Model file for the job. Use its own axes, mm. A direction names the side the tool comes from. Coordinates: 2 decimals unless noted, no trailing zeros. Order: outer loops, then holes, each group sorted by start corner. A loop starts at its lowest first (then second) coordinate and runs counter-clockwise, first axis right, second up.
from build123d import *

# Parameters (mm, degrees)
F0_W     = 38
F0_H     = 69
F0_W_2   = 28
F0_H_2   = 28
F0_H_3   = 1
F0_W_3   = 1
F1_DEPTH = 5
F2_DEPTH = 25
F3_DEPTH = 4
F4_R     = 4.99999


# Not quite as in the source:
# - a fillet or chamfer is up to 0.001 mm smaller than in the source, because OpenCascade refuses the exact size


with BuildPart() as f1:
    # F0 (on Front) → F1 (new body)
    with BuildSketch(Plane.XZ):
        Rectangle(F0_W, F0_H)
        Polygon((-15, 0.5), (-15, 1.5), (-15, 30.5), (15, 30.5), (15, 1.5), (15, 0.5), (15, -0.5), (15, -1.5), (15, -30.5), (-15, -30.5), (-15, -1.5), (-15, -0.5), align=None, mode=Mode.SUBTRACT)
        with Locations((0, 15.5)):
            Rectangle(F0_W_2, F0_H_2)
        with Locations((0, -15.5)):
            Rectangle(F0_W_2, F0_H_2)
        Polygon((-14, -29.5), (-14, -1.5), (-15, -1.5), (-15, -30.5), (15, -30.5), (15, -1.5), (14, -1.5), (14, -29.5), align=None)
        Polygon((-14, 1.5), (-14, 29.5), (14, 29.5), (14, 1.5), (15, 1.5), (15, 30.5), (-15, 30.5), (-15, 1.5), align=None)
        with Locations((0, 1)):
            Rectangle(F0_W_2, F0_H_3)
        with Locations((0, -1)):
            Rectangle(F0_W_2, F0_H_3)
        Rectangle(F0_W_2, F0_H_3)
        with Locations((-14.5, 1)):
            Rectangle(F0_W_3, F0_H_3)
        with Locations((-14.5, 0)):
            Rectangle(F0_W_3, F0_H_3)
        with Locations((-14.5, -1)):
            Rectangle(F0_W_3, F0_H_3)
        with Locations((14.5, 1)):
            Rectangle(F0_W_3, F0_H_3)
        with Locations((14.5, 0)):
            Rectangle(F0_W_3, F0_H_3)
        with Locations((14.5, -1)):
            Rectangle(F0_W_3, F0_H_3)
    extrude(amount=F1_DEPTH)

    # F0 (on Front) → F2 (cut)
    with BuildSketch(Plane.XZ):
        with Locations((0, 15.5)):
            Rectangle(F0_W_2, F0_H_2)
        with Locations((0, -15.5)):
            Rectangle(F0_W_2, F0_H_2)
    extrude(amount=F2_DEPTH, mode=Mode.SUBTRACT)

    # F0 (on Front) → F3 (cut)
    with BuildSketch(Plane.XZ):
        Polygon((-14, 1.5), (-14, 29.5), (14, 29.5), (14, 1.5), (15, 1.5), (15, 30.5), (-15, 30.5), (-15, 1.5), align=None)
        with Locations((14.5, 1)):
            Rectangle(F0_W_3, F0_H_3)
        with Locations((0, 1)):
            Rectangle(F0_W_2, F0_H_3)
        with Locations((-14.5, 1)):
            Rectangle(F0_W_3, F0_H_3)
        Polygon((-14, -29.5), (-14, -1.5), (-15, -1.5), (-15, -30.5), (15, -30.5), (15, -1.5), (14, -1.5), (14, -29.5), align=None)
        with Locations((14.5, -1)):
            Rectangle(F0_W_3, F0_H_3)
        with Locations((0, -1)):
            Rectangle(F0_W_2, F0_H_3)
        with Locations((-14.5, -1)):
            Rectangle(F0_W_3, F0_H_3)
    extrude(amount=F3_DEPTH, mode=Mode.SUBTRACT)

    # F4 (radius 5 in the source; OpenCascade refuses exactly that, so slightly less here)
    f4_edges = [f1.edges().sort_by_distance(p)[0] for p in [
        (-19, -5, 0),
        (0, -5, 34.5),
        (19, -5, 0),
        (0, -5, -34.5),
    ]]
    fillet(f4_edges, radius=F4_R)


solid = f1.part
Q1. Cut at B-B, the plane x = 4.5. Count the separate pieces of the cut face and the enclosed holes in it, plus the area to 3 significant figures.
Established:
separate pieces: 3
enclosed holes: 0
area: 38.3 mm2
Q2. Cut at A-A, the plane y = -3. List the corners of the cut face in (x, z).
Established:
outline: (-18, -33.5) - (18, -33.5) - (18, 33.5) - (-18, 33.5) - close; hole (-15, -30.5) - (15, -30.5) - (15, -0.5) - (-15, -0.5) - close; hole (-15, 0.5) - (15, 0.5) - (15, 30.5) - (-15, 30.5) - close
Q3. Mould opens along X. For faces 3 (the face through (-1, -4, 1)), 4 (the face through (0.27, -3.5, -33.07)), 5 (the face through (17, -4, 0)) say: pulls with the +X half, pulls with the -X half, needs draft (parallel to the pull), parting line crosses it, or undercut.
Established:
face 3: undercut
face 4: needs draft
face 5: pulls with the +X half
Q4. Probe line 1 (Z direction, x = 13, y = -0.35); line 2 (Z direction, x = 4.5, y = -1.3); line 3 (Y direction, x = -6.5, z = 1). List the from-to ranges inside material, lowest first.
Established:
line 1: z = -34.49 to -30.5, -0.5 to 0.5, 30.5 to 34.49
line 2: z = -34.33 to -30.5, -0.5 to 0.5, 30.5 to 34.33
line 3: y = -5 to -4
Q5. Drop flat-ended pins along their axis: P1, Ø1.1, axis at y = -4.5, z = 20, coming from the -X side; P2, Ø0.5, axis at x = -4, y = -4.5, coming from the +Z side; P3, Ø2, axis at y = -2.5, z = -9, coming from the +X side. Give the stop position or say it passes through.
Established:
P1: stops at x = -17.07
P2: stops at z = 32.13
P3: stops at x = 18.77
Q6. Which spindle directions (+Z, -Z, +X, -X, +Y, -Y) get a long thin tool onto all of the face, cutting with end or side? Do faces 1 (the face through (15, -2, 15)), 2 (the face through (0, 0, 0)). Say none if no direction does.
Established:
face 1: +Y
face 2: +Z, -Z, +X, -X, +Y
